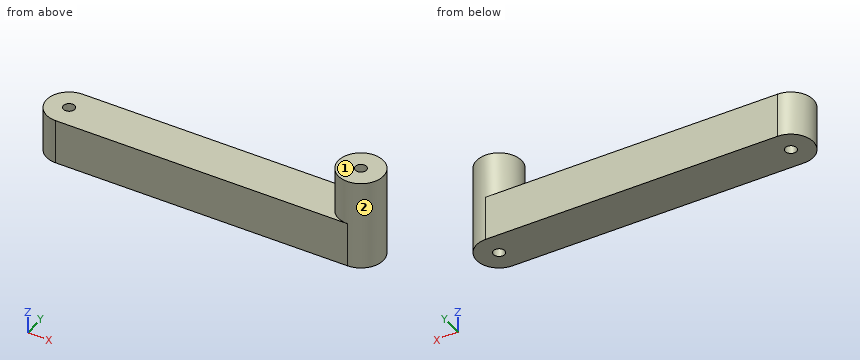
from build123d import *

# Parameters (mm, degrees)
SKETCH_1_R      = 0.5
EXTRUDE_1_DEPTH = 4
SKETCH_2_R      = 2
SKETCH_2_R_2    = 0.5
EXTRUDE_2_DEPTH = 4


with BuildPart() as part:
    # 草图1 → 凸台-拉伸1 (new body)
    with BuildSketch(Plane.XY):
        with BuildLine():
            Line((0, 2), (26, 2))
            ThreePointArc((26, 2), (28, 0), (26, -2))
            Line((26, -2), (0, -2))
            ThreePointArc((0, -2), (-2, 0), (0, 2))
        make_face()
        Circle(SKETCH_1_R, mode=Mode.SUBTRACT)
        with Locations((26, 0)):
            Circle(SKETCH_1_R, mode=Mode.SUBTRACT)
    extrude(amount=EXTRUDE_1_DEPTH)

    # 草图2 → 凸台-拉伸2 (add)
    with BuildSketch(Plane.XY.offset(4)):
        with Locations(Location((26, 0, 0), (0, 0, 90))):
            Circle(SKETCH_2_R)
        with Locations((26, 0)):
            Circle(SKETCH_2_R_2, mode=Mode.SUBTRACT)
    extrude(amount=EXTRUDE_2_DEPTH)


solid = part.part
Input: part model. Units: mm. Frame: model coordinates. Face numbers are marked on the shaded views. A direction names the side the tool comes from. Round coordinates to 2 decimals unless told otherwise and drop trailing zeros. Order: outer loops, then holes, each group sorted by start corner. A loop starts at its lowest first (then second) coordinate and runs counter-clockwise, first axis right, second up.
1. Pin query (flat end, axial travel): P1, Ø2, axis at x = 12, y = 0.5, coming from the +Z side; P2, Ø1.5, axis at x = 24, y = 0.5, coming from the -Z side. Return the tip coordinate at first contact, or that it passes through.
The answers:
P1: stops at z = 4
P2: stops at z = 0
2. Cut plane A-A, the plane y = 0. Output: boundary loops of the cut face in (x, z).
The answers:
outline: (-2, 0) - (-0.5, 0) - (-0.5, 4) - (-2, 4) - close; (0.5, 0) - (25.5, 0) - (25.5, 8) - (24, 8) - (24, 4) - (0.5, 4) - close; (26.5, 0) - (28, 0) - (28, 8) - (26.5, 8) - close
3. Material intervals for line 1 (Y direction, x = 0, z = 1.1); line 2 (Z direction, x = 8.75, y = -1.55); line 3 (X direction, y = 1.65, z = 2), sorted ascending.
The answers:
line 1: y = -2 to -0.5, 0.5 to 2
line 2: z = 0 to 4
line 3: x = -1.13 to 27.13
4. Cut plane C-C, the plane y = -1.2. Output: boundary loops of the cut face in (x, z), then the cut area to 3 significant figures.
The answers:
outline: (-1.6, 0) - (27.6, 0) - (27.6, 8) - (24.4, 8) - (24.4, 4) - (-1.6, 4) - close
area: 130 mm2
5. Set-up query: the marked faces 1 and 2. Return all of +Z, -Z, +X, -X, +Y, -Y with unobstructed straight access to the full face (end or side cutting, diameter ignored); none if empty.
The answers:
face 1: +Z, +X, -X, +Y, -Y
face 2: +Z
6. Cut plane B-B, the plane z = 1.5. Output: boundary loops of the cut face in (x, y).
The answers:
outline: (0, -2) - (26, -2) arc R2 ccw to (26, 2) - (0, 2) arc R2 ccw to start; hole circle Ø1 at (0, 0); hole circle Ø1 at (26, 0)
7. Cut plane D-D, the plane x = 3.5. Output: boundary loops of the cut face in (y, z).
The answers:
outline: (-2, 0) - (2, 0) - (2, 4) - (-2, 4) - close
